Here's how the part is built. I have some questions about the finished solid (model axes, mm). A direction names the side the tool comes from. Give positions to 0.01 mm unless a question says otherwise; leave off trailing zeros. Loops run counter-clockwise (first coordinate to the right, second up) from the corner with the lowest first, then second, coordinate; pieces in that order, holes last. Notation, with made-up numbers: M 89,27 L 94,27 A24 ccw 94,51 Z; hole C 44,-4 d6. An arc over 180 degrees is marked long. Answer as CSV lines item,"result". Start each with the question number.
Item 1: I want a section at B-B on y = 8. List the corners of the cut face in (x, z) for me, plus the area to 3 significant figures.
Item 2: Will these pins go through, and if not, where does the flat tip stop? P1, Ø4, axis at x = 203, y = 6, coming from the -Z side; P2, Ø3.5, axis at x = 153, z = -10, coming from the +Y side; P3, Ø4.5, axis at x = 90, z = -9, coming from the +Y side.
Item 3: If I drill on line 1 along X through (y, z) = (1.45, -9); line 2 along Z through (x, y) = (386, 13.75); line 3 along Y through (x, z) = (169.5, -1.25), over which ranges is the centre line in solid material (lowest first)? Write a range as from..to.
Item 4: For faces 1 (the flat face through (215, 2, -8)), 2 (the flat face through (215, 0, -8)), which set-ups out of +Z, -Z, +X, -X, +Y, -Y let a thin tool reach every point of the face, with its end or its side?
Item 5: I want a section at A-A on x = 98. List the corners of the cut face in (y, z) for me.
from build123d import *

# Parameters (mm, degrees)
EXTRUDE_1_DEPTH     = 436
SKETCH_4_R          = 2.75
CUT_EXTRUDE_3_DEPTH = 2
SKETCH_9_R          = 2.8
CUT_EXTRUDE_8_DEPTH = 437.515750002
CHAMFER_4_SIZE      = 2.098


with BuildPart() as part:
    # Эскиз1 → Бобышка-Вытянуть1 (new body)
    with BuildSketch(Plane(origin=(0, 0, 0), x_dir=(0, 0, -1), z_dir=(1, 0, 0))):
        with BuildLine():
            Line((0, 0), (0, 15))
            Line((0, 15), (1, 15))
            ThreePointArc((1, 15), (1.707106781, 14.707106781), (2, 14))
            Line((2, 14), (2, 3))
            ThreePointArc((2, 3), (2.292893219, 2.292893219), (3, 2))
            Line((3, 2), (14, 2))
            ThreePointArc((14, 2), (14.707106781, 1.707106781), (15, 1))
            Line((15, 1), (15, 0))
            Line((15, 0), (0, 0))
        make_face()
    extrude(amount=EXTRUDE_1_DEPTH)

    # Эскиз4 → Вырез-Вытянуть3 (cut)
    with BuildSketch(Plane.XZ):
        with Locations(Location((372, -9, 0), (0, 0, 270))):
            Circle(SKETCH_4_R)
        with Locations(Location((90, -9, 0), (0, 0, 270))):
            Circle(SKETCH_4_R)
    extrude(amount=-CUT_EXTRUDE_3_DEPTH, mode=Mode.SUBTRACT)

    # Эскиз9 → Вырез-Вытянуть8 (cut, through all)
    with BuildSketch(Plane.XY):
        with Locations((426, 8)):
            Circle(SKETCH_9_R)
        with Locations((10, 8)):
            Circle(SKETCH_9_R)
    extrude(amount=-CUT_EXTRUDE_8_DEPTH, mode=Mode.SUBTRACT)

    # Фаска4
    # the kernel refuses this chamfer: 2.098 mm, written as the material it takes off along each edge
    with BuildSketch(Plane(origin=(10, 8, 0), x_dir=(1, 0, 0), z_dir=(0, -1, 0))) as chamfer_4_piece_1:
        Polygon((2.8 + CHAMFER_4_SIZE, 0), (2.8, -CHAMFER_4_SIZE), (2.8, 0), align=None)
    revolve(axis=Axis((10, 8, 0), (0, 0, 1)), mode=Mode.SUBTRACT)
    with BuildSketch(Plane(origin=(426, 8, 0), x_dir=(1, 0, 0), z_dir=(0, -1, 0))) as chamfer_4_piece_2:
        Polygon((2.8 + CHAMFER_4_SIZE, 0), (2.8, -CHAMFER_4_SIZE), (2.8, 0), align=None)
    revolve(axis=Axis((426, 8, 0), (0, 0, 1)), mode=Mode.SUBTRACT)


solid = part.part
Result:
1,outline,"M 0,-2 L 7.1,-2 L 5.1,0 L 0,0 Z; M 12.9,-2 L 423.1,-2 L 421.1,0 L 14.9,0 Z; M 428.9,-2 L 436,-2 L 436,0 L 430.9,0 Z"
1,area,"841 mm^2"
2,P1,"z = -2"
2,P2,"y = 2"
2,P3,"through"
3,line 1,"0..87.25, 92.75..369.25, 374.75..436"
3,line 2,"-2..0"
3,line 3,"0..14.97"
4,face 1,"-Z, +X, -X, +Y"
4,face 2,"+Z, -Z, +X, -X, -Y"
5,outline,"M 0,-15 L 1,-15 A1 ccw 2,-14 L 2,-3 A1 cw 3,-2 L 14,-2 A1 ccw 15,-1 L 15,0 L 0,0 Z"
